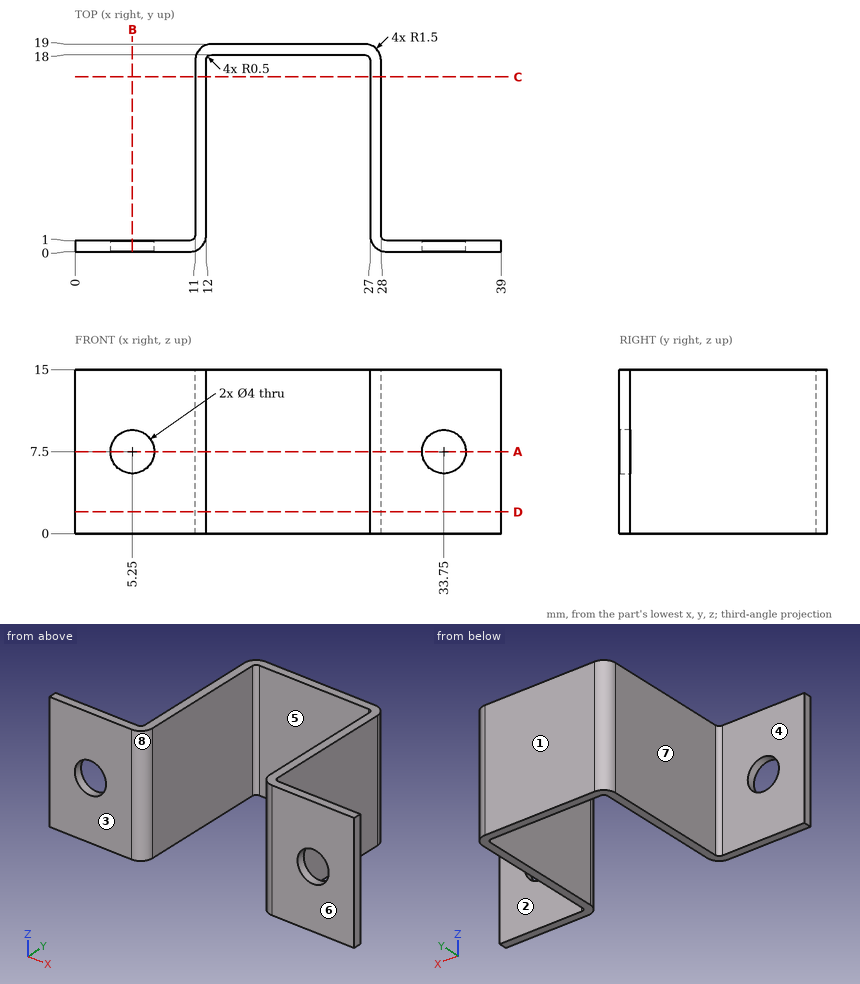
Drawing for the job (mm, zero at the part's lowest x, y, z). A direction names the side the tool comes from. Coordinates: 2 decimals unless noted, no trailing zeros. Order: outer loops, then holes, each group sorted by start corner. A loop starts at its lowest first (then second) coordinate and runs counter-clockwise, first axis right, second up. Notation, with made-up numbers: (80.5, -38) -> (91.5, -38) arc R32 ccw to (91.5, -7) -> close; hole circle Ø3 at (-36.5, -30.75). An arc over 180 degrees is marked (long way). Return JSON: item names as keys, results as strings.
Item 1: Wall check: line 1 along X through (y, z) = (14, 1.75); line 2 along X through (y, z) = (0.3, 7.5); line 3 along Y through (x, z) = (26, 3.5). Give the ranges that are in metal, low to high. Write a range as from..to.
Model answer:
{"line 1": "x = 11..12, 27..28", "line 2": "x = 0..3.25, 7.25..11.4, 27.6..31.75, 35.75..39", "line 3": "y = 18..19"}
Item 2: Slice it at C-C (y = 16). Write the cut outline in (x, z).
Model answer:
{"outline": "(11, 0) -> (12, 0) -> (12, 15) -> (11, 15) -> close; (27, 0) -> (28, 0) -> (28, 15) -> (27, 15) -> close"}
Item 3: Slice it at B-B (x = 5.25). Write the cut outline in (y, z), then the cut area to 3 significant figures.
Model answer:
{"outline": "(0, 0) -> (1, 0) -> (1, 5.5) -> (0, 5.5) -> close; (0, 9.5) -> (1, 9.5) -> (1, 15) -> (0, 15) -> close", "area": "11.0 mm²"}
Item 4: Mould opens along X. For the marked faces 6, 7 and 8 say: pulls with the +X half, pulls with the -X half, needs draft (parallel to the pull), parting line crosses it, or undercut.
Model answer:
{"face 6": "needs draft", "face 7": "pulls with the -X half", "face 8": "undercut"}
Item 5: Slice it at A-A (z = 7.5). Write the cut outline in (x, y), then the cut area to 3 significant figures.
Model answer:
{"outline": "(0, 0) -> (3.25, 0) -> (3.25, 1) -> (0, 1) -> close; (7.25, 0) -> (10.5, 0) arc R1.5 ccw to (12, 1.5) -> (12, 17.5) arc R0.5 cw to (12.5, 18) -> (26.5, 18) arc R0.5 cw to (27, 17.5) -> (27, 1.5) arc R1.5 ccw to (28.5, 0) -> (31.75, 0) -> (31.75, 1) -> (28.5, 1) arc R0.5 cw to (28, 1.5) -> (28, 17.5) arc R1.5 ccw to (26.5, 19) -> (12.5, 19) arc R1.5 ccw to (11, 17.5) -> (11, 1.5) arc R0.5 cw to (10.5, 1) -> (7.25, 1) -> close; (35.75, 0) -> (39, 0) -> (39, 1) -> (35.75, 1) -> close", "area": "65.3 mm²"}
Item 6: Pin check, flat tips, straight feed: P1, Ø4.5, axis at y = 9, z = 4.5, coming from the +X side; P2, Ø1, axis at x = 27, z = 9.5, coming from the -Y side; P3, Ø8.5, axis at x = 5.5, z = 8, coming from the +Y side. Stop position of each tip, or through.
Model answer:
{"P1": "stops at x = 28", "P2": "stops at y = 0.38", "P3": "stops at y = 1"}
Item 7: 3-axis set-ups, long thin cutter, end or side, ignore diameter. For the marked faces 1, 2, 3, 4 and 5: which of +Z, -Z, +X, -X, +Y, -Y reach the whole face in a straight line?
Model answer:
{"face 1": "+Z, -Z, +X, -X, +Y", "face 2": "+Z, -Z, +X, +Y", "face 3": "+Z, -Z, +X, -X, -Y", "face 4": "+Z, -Z, -X, +Y", "face 5": "+Z, -Z, -Y"}
Item 8: Slice it at D-D (z = 2). Write the cut outline in (x, y).
Model answer:
{"outline": "(0, 0) -> (10.5, 0) arc R1.5 ccw to (12, 1.5) -> (12, 17.5) arc R0.5 cw to (12.5, 18) -> (26.5, 18) arc R0.5 cw to (27, 17.5) -> (27, 1.5) arc R1.5 ccw to (28.5, 0) -> (39, 0) -> (39, 1) -> (28.5, 1) arc R0.5 cw to (28, 1.5) -> (28, 17.5) arc R1.5 ccw to (26.5, 19) -> (12.5, 19) arc R1.5 ccw to (11, 17.5) -> (11, 1.5) arc R0.5 cw to (10.5, 1) -> (0, 1) -> close"}
